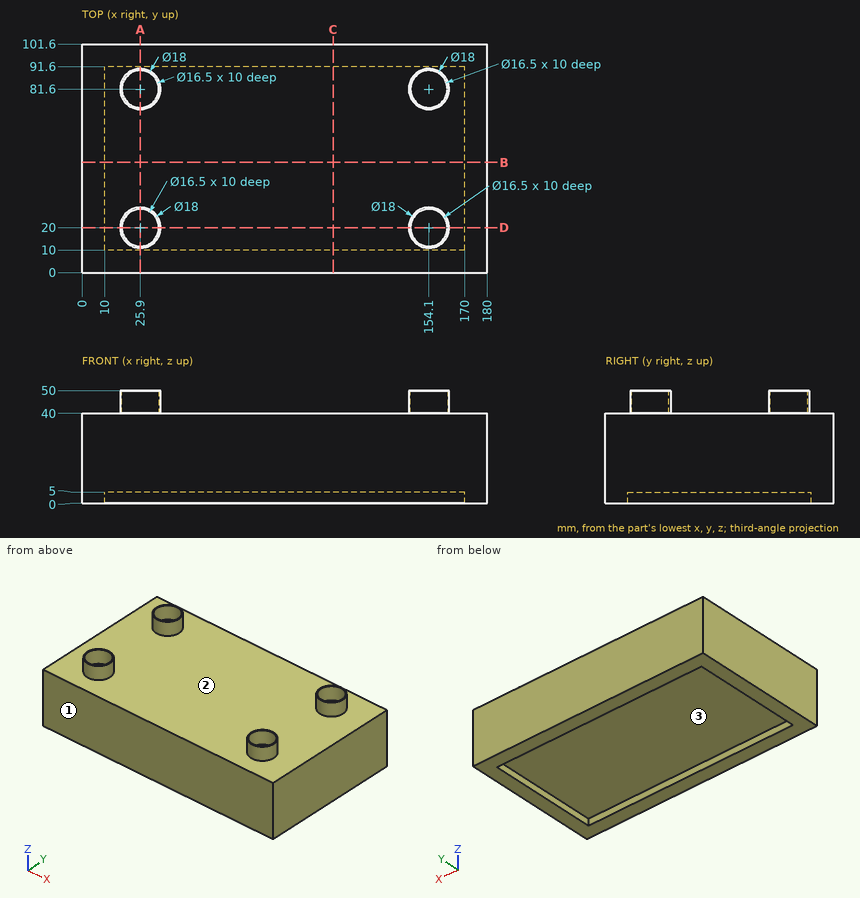
Geometry check sheet. Reference: drawing and pictorial views, mm from the part's lowest x, y, z. A direction names the side the tool comes from. Give positions to 0.01 mm unless a question says otherwise; leave off trailing zeros. Write each loop counter-clockwise with the first axis right and the second up, starting at its lowest first coordinate (ties: lowest second). Pieces come first, ordered by that corner, then holes.
Item 1: Cross-section at C-C (x = 111.5). Enter the section's corners in (y, z), and give its area (3 significant figures).
Item 2: Cross-section at D-D (y = 20). Enter the section's corners in (x, z).
Item 3: Access from +Z, -Z, +X, -X, +Y, -Y to the whole of each face (thin tool, end or side, straight path). Record for the marked faces 1, 2 and 3.
Item 4: Gauge pin test, flat ends, axial feed: pin 1 (15 mm diameter, centred on x = 154.1, y = 20, fed in from +Z); pin 2 (24.5 mm diameter, centred on x = 68, y = 54.5, fed in from -Z). Record the tip position at first contact, or that the pin passes through.
Item 5: Cross-section at A-A (x = 25.9). Enter the section's corners in (y, z).
Item 6: Scan lines: L1, parallel to Y at x = 154.1, z = 47.5; L2, parallel to Z at x = 72, y = 22.5; L3, parallel to Z at x = 45, y = 95. Record each from-to range of solid material in increasing order.
Item 7: Cross-section at B-B (y = 49). Enter the section's corners in (x, z).
Report:
1. outline: (0, 0) - (10, 0) - (10, 5) - (91.6, 5) - (91.6, 0) - (101.6, 0) - (101.6, 40) - (0, 40) - close
1. area: 3,660 mm2
2. outline: (0, 0) - (10, 0) - (10, 5) - (170, 5) - (170, 0) - (180, 0) - (180, 40) - (163.1, 40) - (163.1, 50) - (162.35, 50) - (162.35, 40) - (145.85, 40) - (145.85, 50) - (145.1, 50) - (145.1, 40) - (34.9, 40) - (34.9, 50) - (34.15, 50) - (34.15, 40) - (17.65, 40) - (17.65, 50) - (16.9, 50) - (16.9, 40) - (0, 40) - close
3. face 1: +Z, -Z, +X, -X, -Y
3. face 2: +Z
3. face 3: -Z
4. pin 1: stops at z = 40
4. pin 2: stops at z = 5
5. outline: (0, 0) - (10, 0) - (10, 5) - (91.6, 5) - (91.6, 0) - (101.6, 0) - (101.6, 40) - (90.6, 40) - (90.6, 50) - (89.85, 50) - (89.85, 40) - (73.35, 40) - (73.35, 50) - (72.6, 50) - (72.6, 40) - (29, 40) - (29, 50) - (28.25, 50) - (28.25, 40) - (11.75, 40) - (11.75, 50) - (11, 50) - (11, 40) - (0, 40) - close
6. L1: y = 11 to 11.75, 28.25 to 29, 72.6 to 73.35, 89.85 to 90.6
6. L2: z = 5 to 40
6. L3: z = 0 to 40
7. outline: (0, 0) - (10, 0) - (10, 5) - (170, 5) - (170, 0) - (180, 0) - (180, 40) - (0, 40) - close
